Verification items for the finished model (mm, model axes). Coordinates: 2 decimals unless noted, no trailing zeros. Order: outer loops, then holes, each group sorted by start corner. A loop starts at its lowest first (then second) coordinate and runs counter-clockwise, first axis right, second up. Notation, with made-up numbers: (-35.5, 24.25) -> (-14.5, 24.25) arc R22 ccw to (-14.5, 34.25) -> close; hole circle Ø4 at (-5.75, -14.5). An arc over 180 degrees is marked (long way). Write item = value, one per line. Start each with the question number.
1. Thickness scan on line 1 along Y through (x, z) = (4, 0.75); line 2 along Y through (x, z) = (82, 0.55); line 3 along X through (y, z) = (52, 0.75). Record the ranges inside material, lowest first. Write a range as from..to.
2. Go/stop test with a flat-tipped pin: P1, Ø2, axis at x = -36, y = 65, coming from the -Z side. Record where the tip stops, or that it passes through.
3. Cross-section at C-C on y = -73. Record the cut outline in (x, z), plus the area to 3 significant figures.
4. Cross-section at A-A on z = 0.4. Record the cut outline in (x, y), plus the area to 3 significant figures.
5. Cross-section at B-B on x = -102.5. Record the cut outline in (y, z).
Autodesk Fusion 360 part; units mm, degrees
sketch "Round Bed" plane through (0, 0, 0) normal (0, 0, 1) x (1, 0, 0)
  line L0 (-90.1561, -90.1561) -> (90.1561, -90.1561) construction
  line L1 (90.1561, -90.1561) -> (90.1561, 90.1561) construction
  line L2 (90.1561, 90.1561) -> (-90.1561, 90.1561) construction
  line L3 (-90.1561, 90.1561) -> (-90.1561, -90.1561) construction
  line L4 (-90.1561, -90.1561) -> (90.1561, 90.1561) construction
  line L5 (90.1561, -90.1561) -> (-90.1561, 90.1561) construction
  line L6 (-31.875, -137.5) -> (31.875, -137.5)
  line L7 (0, 0) -> (0, -137.5) construction
  arc A0 (-42.0024, -127.3726) -> (-31.875, -137.5) centre (-31.875, -127.3726) ccw
  arc A1 (-42.0024, -127.3726) -> (-48.2938, -117.9998) centre (-52.1298, -127.3726) ccw
  arc A2 (31.875, -137.5) -> (42.0024, -127.3726) centre (31.875, -127.3726) ccw
  arc A3 (48.2938, -117.9998) -> (42.0024, -127.3726) centre (52.1298, -127.3726) ccw
  circle A4 centre (-31.875, -127.3726) radius 2
  circle A5 centre (31.875, -127.3726) radius 2
  arc A6 (48.2938, -117.9998) -> (-48.2938, -117.9998) centre (0, 0) ccw
  dimension "d4" = 255
  dimension "d6" = 63.75
  dimension "d7" = 137.5
  dimension "d10" = 4
sketch "Square Bed" plane through (0, 0, 0) normal (0, 0, 1) x (1, 0, 0)
  line L0 (-90, -90) -> (90, 90) construction
  line L1 (90, -90) -> (-90, 90) construction
  line L2 (-31.8198, -137.2792) -> (31.8198, -137.2792)
  line L3 (90, -90) -> (90, 90) construction
  arc A0 (48.2308, -117.7871) -> (41.9434, -127.1557) centre (52.0669, -127.1557) ccw
  arc A1 (48.2308, -117.7871) -> (-48.2308, -117.7871) centre (0, 0) ccw
  line L4 (-90, 90) -> (-90, -90) construction
  arc A2 (-41.9434, -127.1557) -> (-48.2308, -117.7871) centre (-52.0669, -127.1557) ccw
  arc A3 (-41.9434, -127.1557) -> (-31.8198, -137.2792) centre (-31.8198, -127.1557) ccw
  line L5 (-90, -90) -> (90, -90) construction
  line L6 (90, 90) -> (-90, 90) construction
  circle A4 centre (-31.8198, -127.1557) radius 2
  arc A5 (31.8198, -137.2792) -> (41.9434, -127.1557) centre (31.8198, -127.1557) ccw
  circle A6 centre (31.8198, -127.1557) radius 2
  line L7 (0, 0) -> (0, -137.2792) construction
  dimension "d14" = 63.6396
  dimension "d16" = 4
  dimension "d17" = 180
  dimension "d18" = 127.2792
  dimension "d20" = 137.2792
extrude "Round Bed" [suppressed]
extrude "Square Bed (1)" add sketch "Square Bed" along normal blind 1
equation "d4 = Round_Bed_Size"
equation "d6 = d4 / 4"
equation "d7 = d4 / 2 + 10 mm"
equation "Round_Bed_Size = 255 mm"
equation "Square_Bed_Size = 180 mm"
equation "d14 = ( d18 * 2 ) / 4"
equation "d17 = Square_Bed_Size"
equation "d20 = d18 + 10 mm"
properties part number "180mm Square Bed"
Worked out:
q1.line_1 = -137.28..127.22
q1.line_2 = -97.34..97.34
q1.line_3 = -116.17..116.17
q2.P1 = 0
q3.outline = (-104.26, 0) -> (104.26, 0) -> (104.26, 1) -> (-104.26, 1) -> close
q3.area = 209 mm²
q4.outline = (-48.23, -117.79) arc R10.12 cw to (-41.94, -127.16) arc R10.12 ccw to (-31.82, -137.28) -> (31.82, -137.28) arc R10.12 ccw to (41.94, -127.16) arc R10.12 cw to (48.23, -117.79) arc R127.28 ccw (long way) to start; hole circle Ø4 at (-31.82, -127.16); hole circle Ø4 at (31.82, -127.16)
q4.area = 51,900 mm²
q5.outline = (-75.46, 0) -> (75.46, 0) -> (75.46, 1) -> (-75.46, 1) -> close
